For this review, use the dimensioned drawing (mm, ordinates from the lowest corner) and the shaded views. A direction names the side the tool comes from. Give positions to 0.01 mm unless a question says otherwise; leave off trailing zeros. Loops run counter-clockwise (first coordinate to the right, second up) from the corner with the lowest first, then second, coordinate; pieces in that order, holes last. Notation, with made-up numbers: (-26.5, -24) - (25.5, -24) arc R5 ccw to (25.5, -17) - close; hole circle Ø5 at (71.5, 38). An arc over 180 degrees is marked (long way). Put each result on its own line as item: value.
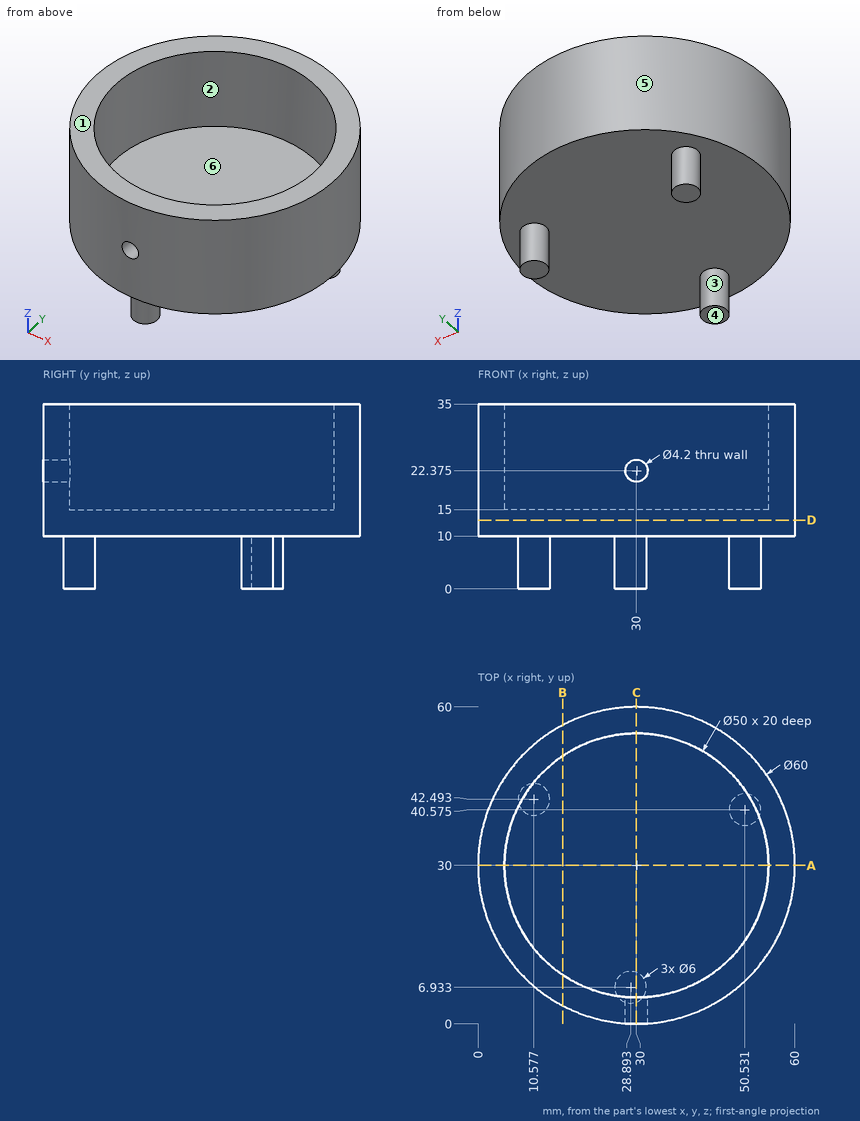
1) Wall thickness on line 1 (Y direction, x = 30, z = 26); line 2 (Z direction, x = 30, y = 2) (1 decimal); line 3 (Z direction, x = 17, y = 10.5): over which ranges is each line inside the solid? List them lowest first.
Geometry check:
line 1: y = 0 to 5, 55 to 60
line 2: z = 10 to 20.3, 24.5 to 35
line 3: z = 10 to 15
2) Take a section at B-B on x = 16. State the section outline as (y, z) points, and give its area (3 significant figures).
Geometry check:
outline: (3.47, 10) - (56.53, 10) - (56.53, 35) - (50.71, 35) - (50.71, 15) - (9.29, 15) - (9.29, 35) - (3.47, 35) - close
area: 498 mm²
3) Draft analysis for pull direction X (two halves, no side actions). For the marked faces 4, 5 and 6, state which applies: pulls with the +X half, pulls with the -X half, needs draft (parallel to the pull), parting line crosses it, or undercut.
Geometry check:
face 4: needs draft
face 5: parting line crosses it
face 6: undercut
4) Take a section at C-C on x = 30. State the section outline as (y, z) points (1 decimal), and give its area (3 significant figures).
Geometry check:
outline: (0, 10) - (4.1, 10) - (4.1, 0) - (9.7, 0) - (9.7, 10) - (60, 10) - (60, 35) - (55, 35) - (55, 15) - (5, 15) - (5, 20.3) - (0, 20.3) - close; (0, 24.5) - (5, 24.5) - (5, 35) - (0, 35) - close
area: 535 mm²
5) For the marked faces 1, 2 and 3, list the 3-axis set-ups (+Z, -Z, +X, -X, +Y, -Y) from which the entire face can be reached by the end or side of a thin tool; tool diameter is ignored.
Geometry check:
face 1: +Z, +X, -X, +Y, -Y
face 2: +Z
face 3: -Z
6) Take a section at D-D on z = 13. State the section outline as (x, y) points.
Geometry check:
outline: circle Ø60 at (30, 30)
7) Take a section at A-A on y = 30. State the section outline as (x, z) points, and give its area (3 significant figures).
Geometry check:
outline: (0, 10) - (60, 10) - (60, 35) - (55, 35) - (55, 15) - (5, 15) - (5, 35) - (0, 35) - close
area: 500 mm²
8) Insertion check: pin 1 Ø8 at (x, y) = (37, 27.5) entering from +Z; pin 2 Ø5 at (y, z) = (44.5, 20) entering from +X (1 decimal); pin 3 Ø8 at (x, y) = (34.5, 18.5) entering from -Z. Each pin has a flat end and moves straight along its axis. Give the tip position at first contact, or say it passes through.
Geometry check:
pin 1: stops at z = 15
pin 2: stops at x = 57.5
pin 3: stops at z = 10
